Autodesk Inventor part; units mm, degrees
ref_plane "YZ Plane" through (0, 0, 0) normal (1, 0, 0) x (0, 1, 0)
ref_plane "XZ Plane" through (0, 0, 0) normal (0, 1, 0) x (-1, 0, 0)
ref_plane "XY Plane" through (0, 0, 0) normal (0, 0, 1) x (1, 0, 0)
sketch "Sketch1" plane through (0, 0, 0) normal (1, 0, 0) x (0, 1, 0)
  line L0 (0, 0) -> (0, -2.5116) construction
  line L1 (0, 0) -> (2.3876, 0)
  line L2 (2.3876, 0) -> (2.3876, 1.524)
  line L3 (2.3876, 1.524) -> (2.54, 1.524)
  line L4 (2.54, 1.524) -> (2.54, 2.413)
  line L5 (2.54, 2.413) -> (1.651, 2.413)
  line L6 (1.651, 2.413) -> (1.651, 4.445)
  line L7 (1.651, 4.445) -> (2.54, 4.445)
  line L8 (2.54, 4.445) -> (2.54, 5.334)
  line L9 (2.54, 5.334) -> (1.9685, 5.334)
  line L10 (1.9685, 5.334) -> (1.9685, 11.684)
  line L11 (1.9685, 11.684) -> (0.6985, 11.684)
  line L12 (0.6985, 11.684) -> (0.4445, 20.574)
  line L13 (0.4445, 20.574) -> (0, 20.574)
  line L14 (0, 20.574) -> (0, 0)
  dimension "d0" = 4.7752
  dimension "d2" = 5.08
  dimension "d3" = 3.302
  dimension "d4" = 3.937
  dimension "d5" = 1.397
  dimension "d6" = 0.889
  dimension "d7" = 1.524
  dimension "d8" = 2.413
  dimension "d9" = 4.445
  dimension "d10" = 5.334
  dimension "d11" = 11.684
  dimension "d12" = 20.574
revolve "Revolution1" add sketch "Sketch1" angle 360 about axis through (0, 0, 0) along (0, 0, -1)
sketch "Sketch2" plane through (0, 0, 0) normal (0, 0, -1) x (-1, 0, 0)
  circle A0 centre (0, 0) radius 2.3876
  line L0 (-0.4445, 2.3876) -> (0.4445, 2.3876)
  line L1 (0.4445, 2.3876) -> (0.4445, -2.3876)
  line L2 (0.4445, -2.3876) -> (-0.4445, -2.3876)
  line L3 (-0.4445, -2.3876) -> (-0.4445, 2.3876)
  dimension "d14" = 0.889
  dimension "d16" = 0.4445
extrude "Extrusion1" cut sketch "Sketch2" against normal blind 1.524 contours L1 A0 L3 | A0 L0 L1 | L1 L2 A0 | A0 L3 L0 | L2 L3 A0
thread "Thread1"
equation "\"d16\" = 0.5 * d14"
properties part number "Fuel Intake Adjuster Pin"
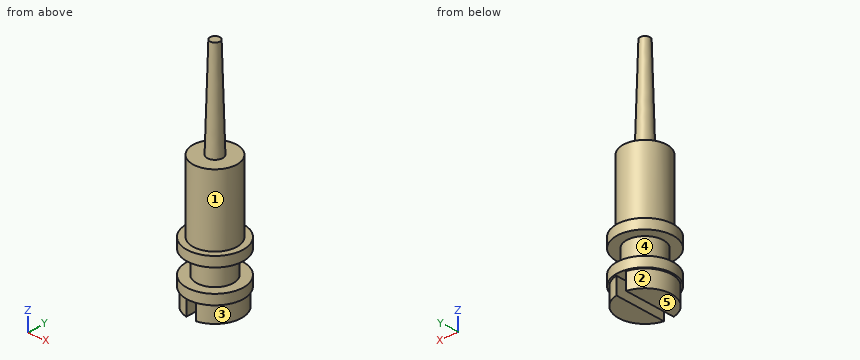
Source: CAD feature listing. Evaluate the final solid. Frame: model axes, mm. Face numbers are marked on the shaded views. A direction names the side the tool comes from. Give positions to 0.01 mm unless a question says otherwise; leave off trailing zeros. Loops run counter-clockwise (first coordinate to the right, second up) from the corner with the lowest first, then second, coordinate; pieces in that order, holes last. Notation, with made-up numbers: M 24,53 L 78,53 A23 cw 78,90 Z; hole C -1,-13 d6. An arc over 180 degrees is marked long. Put each result on its own line as item: value.
Q1. Line query: probe 1 along Z at (x, y) = (-1.95, -0.9) (3 decimals); probe 2 along Z at (x, y) = (1.75, -0.65) (3 decimals); probe 3 along X at (y, z) = (0.1, 3.5). Output: solid intervals per line, ascending. Write a range as [from, to].
Response values:
probe 1: z = [0, 2.413], [4.445, 5.334]
probe 2: z = [0, 2.413], [4.445, 11.684]
probe 3: x = [-1.65, 1.65]
Q2. Section A-A (x = 2.2). Return the cut outline in (y, z) (3 decimals), and give its area (3 significant figures).
Response values:
outline: M -1.269,1.524 L -0.928,1.524 L -0.928,0 L 0.928,0 L 0.928,1.524 L 1.269,1.524 L 1.269,2.413 L -1.269,2.413 Z; M -1.269,4.445 L 1.269,4.445 L 1.269,5.334 L -1.269,5.334 Z
area: 7.34 mm²
Q3. Section B-B (x = 0). Return the cut outline in (y, z) (1 decimal).
Response values:
outline: M -2.5,1.5 L 2.5,1.5 L 2.5,2.4 L 1.7,2.4 L 1.7,4.4 L 2.5,4.4 L 2.5,5.3 L 2,5.3 L 2,11.7 L 0.7,11.7 L 0.4,20.6 L -0.4,20.6 L -0.7,11.7 L -2,11.7 L -2,5.3 L -2.5,5.3 L -2.5,4.4 L -1.7,4.4 L -1.7,2.4 L -2.5,2.4 Z
Q4. Section D-D (z = 9.5). Return the cut outline in (x, y).
Response values:
outline: C 0,0 d3.94
Q5. Pin query (flat end, axial travel): P1, Ø1, axis at x = 0, z = 13, coming from the +Y side; P2, Ø1, axis at y = 0.5, z = 18, coming from the -X side; P3, Ø0.5, axis at y = -1, z = 1, coming from the -X side. Return the tip coordinate at first contact, or that it passes through.
Response values:
P1: stops at y = 0.68
P2: stops at x = -0.52
P3: stops at x = -2.27
Q6. Reachability of the marked faces 1, 2, 3, 4 and 5 from +Z, -Z, +X, -X, +Y, -Y: full face, straight path, thin tool, end or side. Return the list, or none.
Response values:
face 1: +Z
face 2: -Z, -X
face 3: -Z, +X
face 4: none
face 5: -Z, +X, -X, +Y, -Y
